from build123d import *

# Parameters (mm, degrees)
FILLET1_R          = 1.524
SKETCH4_R          = 8.89
CUT_EXTRUDE1_DEPTH = 5.08
FILLET2_R          = 5.08


with BuildPart() as part:
    # Sketch3 → Revolve1 (revolve)
    with BuildSketch(Plane.XY, mode=Mode.PRIVATE) as revolve1_sk:
        with BuildLine():
            Line((0, 0), (12.7, 0))
            Line((12.7, 0), (25.4, 59.10038719))
            Line((25.4, 59.10038719), (22.140333333, 59.10038719))
            Line((22.140333333, 59.10038719), (9.228066554, 16.982885))
            ThreePointArc((9.228066554, 16.982885), (5.738226469, 12.050952327), (0, 10.16))
            Line((0, 10.16), (0, 0))
        make_face()
    revolve(revolve1_sk.sketch.rotate(Axis((0, 0, 0), (0, 1, 0)), 90), axis=Axis((0, 0, 0), (0, 1, 0)))

    # Fillet1
    fillet1_edges = [part.edges().sort_by_distance(p)[0] for p in [
        (0, 59.10038719, 25.4),
        (0, 59.10038719, 22.140333333),
    ]]
    fillet(fillet1_edges, radius=FILLET1_R)

    # Sketch4 → Cut-Extrude1 (cut)
    with BuildSketch(Plane.XZ):
        with Locations(Location((0, 0, 0), (0, 0, 270))):
            Circle(SKETCH4_R)
    extrude(amount=-CUT_EXTRUDE1_DEPTH, mode=Mode.SUBTRACT)

    # Fillet2
    fillet2_edges = [part.edges().sort_by_distance(p)[0] for p in [
        (0, 5.08, 8.89),
    ]]
    fillet(fillet2_edges, radius=FILLET2_R - 0.0001)  # a hair under: the kernel refuses the full size


solid = part.part
Could you check a few things on this model? Use its own coordinates, in mm. Give positions to 0.01 mm unless a question says otherwise; leave off trailing zeros. Loops run counter-clockwise (first coordinate to the right, second up) from the corner with the lowest first, then second, coordinate; pieces in that order, holes last. Notation, with made-up numbers: M 6.5,-20 L 19.5,-20 A12 cw 19.5,0 Z; hole C -1.5,57 d1. An arc over 180 degrees is marked long. Answer as a JSON object with one key per item and string values.
Q1. If I drill on probe 1 along X at (y, z) = (0.05, 0); probe 2 along Z at (x, y) = (8, 19); probe 3 along X at (y, z) = (37.5, 8), over which ranges is the centre line in solid material (lowest first)? Write a range as [from, to].
Values found:
{"probe 1": "x = [-12.71, -8.89], [8.89, 12.71]", "probe 2": "z = [-14.75, -5.74], [5.74, 14.75]", "probe 3": "x = [-19.15, -13.3], [13.3, 19.15]"}
Q2. If we mould it in two halves opening along Z, with no side actions, what happens to faces 1 (the flat face through (3, 0, -9)), 2 (the conical face through (13.7, 32.66, 3.04)), 3 (the conical face through (15.6, 22.7, -8.1))? For each: pulls with the +Z half, pulls with the -Z half, needs draft (parallel to the pull), parting line crosses it, or undercut.
Values found:
{"face 1": "needs draft", "face 2": "undercut", "face 3": "parting line crosses it"}
Q3. Suppose I cut it at A-A, the plane y = 46.5. List the corners of the cut face in (x, z) for me, plus the area to 3 significant figures.
Values found:
{"outline": "C 0,0 d45.38; hole C 0,0 d36.55", "area": "568 mm²"}
Q4. For P1, Ø10, axis at y = 50.5, z = 13.5, coming from the +X side; P2, Ø12, axis at y = 42.5, z = 8.5, coming from the -X side; P3, Ø10, axis at x = -12, z = -14.5, coming from the +Y side; P4, Ø6, axis at y = 7, z = 10.5, coming from the +X side, each with a flat end and sliding along its axis, tell me the tip position at first contact or that it passes through.
Values found:
{"P1": "stops at x = 22.28", "P2": "stops at x = -22.35", "P3": "stops at y = 59.1", "P4": "stops at x = 12.21"}
Q5. Suppose I cut it at B-B, the plane y = 29.5. List the corners of the cut face in (x, z) for me.
Values found:
{"outline": "C 0,0 d38.08; hole C 0,0 d26.13"}
